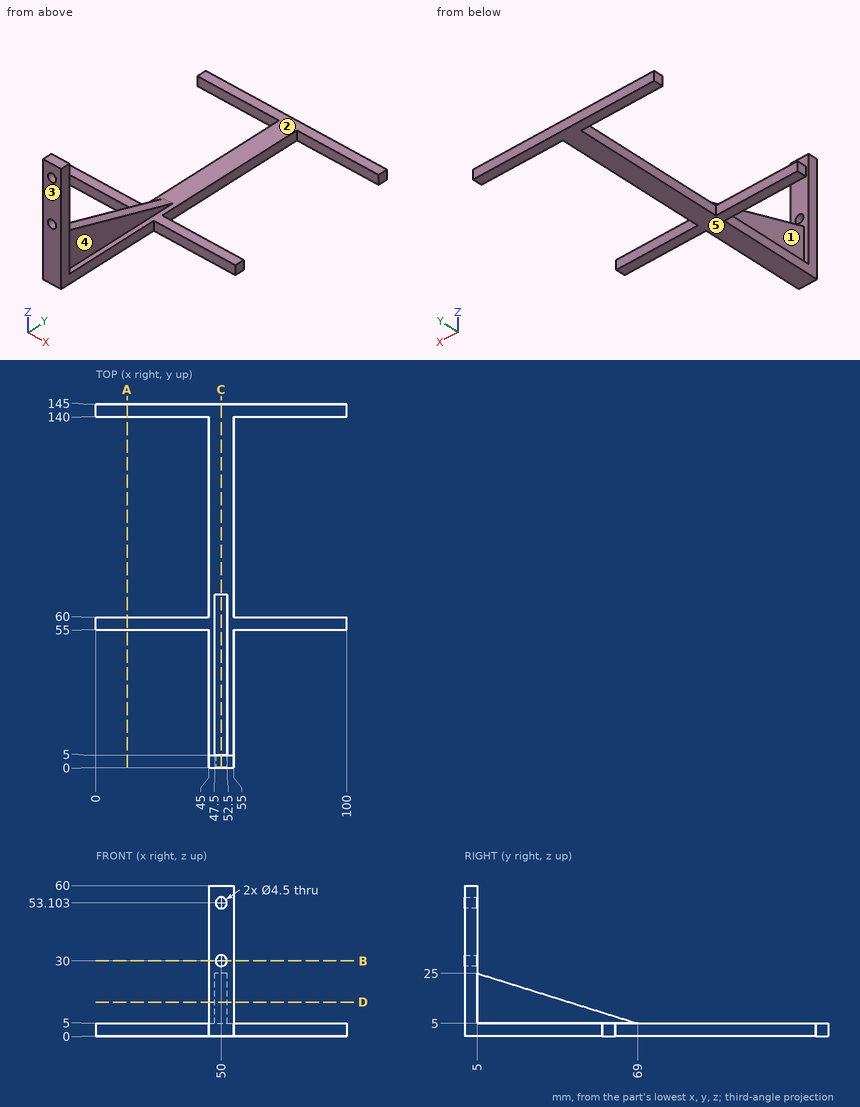
Answer from the drawing. Dimensions are ordinates in mm from the lowest x, y and z of the part. A direction names the side the tool comes from. Give positions to 0.01 mm unless a question says otherwise; leave off trailing zeros. Loops run counter-clockwise (first coordinate to the right, second up) from the corner with the lowest first, then second, coordinate; pieces in that order, holes last.
Item 1: Find the intervals of material crossed by line 1 along Z through (x, y) = (50, 3.85); line 2 along X through (y, z) = (3.2, 30); line 3 along Y through (x, z) = (89, 3.5), in increasing order.
Derived:
line 1: z = 0 to 27.75, 32.25 to 50.85, 55.35 to 60
line 2: x = 45 to 47.75, 52.25 to 55
line 3: y = 55 to 60, 140 to 145
Item 2: A tool of negligible diameter and unlimited length cuts with its end or side. For the marked faces 1, 2, 3, 4 and 5, from which of +Z, -Z, +X, -X, +Y, -Y can it reach the whole face along a straight path? Write none if from no direction.
Derived:
face 1: +Z, -X, +Y
face 2: +Z, +Y
face 3: +Z, -Z, +X, -X, -Y
face 4: +Z, +X, +Y
face 5: -Z, +X, -X, +Y, -Y
Item 3: A cutting plane is placed at D-D (z = 13.5). Give the vertices of the cut face in (x, y).
Derived:
outline: (45, 0) - (55, 0) - (55, 5) - (52.5, 5) - (52.5, 41.8) - (47.5, 41.8) - (47.5, 5) - (45, 5) - close
Item 4: A cutting plane is placed at B-B (z = 30). Give the vertices of the cut face in (x, y).
Derived:
outline: (45, 0) - (47.75, 0) - (47.75, 5) - (45, 5) - close; (52.25, 0) - (55, 0) - (55, 5) - (52.25, 5) - close
Item 5: A cutting plane is placed at A-A (x = 12.5). Give the vertices of the cut face in (y, z).
Derived:
outline: (55, 0) - (60, 0) - (60, 5) - (55, 5) - close; (140, 0) - (145, 0) - (145, 5) - (140, 5) - close
Item 6: A cutting plane is placed at C-C (x = 50). Give the vertices of the cut face in (y, z), then the cut area to 4 significant figures.
Derived:
outline: (0, 0) - (145, 0) - (145, 5) - (69, 5) - (5, 25) - (5, 27.75) - (0, 27.75) - close; (0, 32.25) - (5, 32.25) - (5, 50.85) - (0, 50.85) - close; (0, 55.35) - (5, 55.35) - (5, 60) - (0, 60) - close
area: 1,595 mm2
Item 7: Each of these flat-tipped pins is pushed along its axis until it touches: pin 1 Ø6 at (x, z) = (50, 53.1) entering from -Y; pin 2 Ø2 at (y, z) = (25.5, 18.5) entering from +X; pin 3 Ø1.5 at (x, z) = (88, 3) entering from -Y; pin 4 Ø16 at (y, z) = (43, 11.5) entering from -X. Where does it stop, or does it pass through?
Derived:
pin 1: stops at y = 0
pin 2: stops at x = 52.5
pin 3: stops at y = 55
pin 4: stops at x = 45
